The model under review builds one solid part; all positions refer to its coordinate system, in mm. Face numbers are marked on the shaded views. Round coordinates to 2 decimals unless told otherwise and drop trailing zeros. Order: outer loops, then holes, each group sorted by start corner. A loop starts at its lowest first (then second) coordinate and runs counter-clockwise, first axis right, second up. Notation, with made-up numbers: (37, 57.5) -> (51, 57.5) arc R12 cw to (51, 67.5) -> close; hole circle Ø6 at (63.5, 76). An arc over 180 degrees is marked (long way). Return JSON: item names as keys, results as strings. Group by question number.
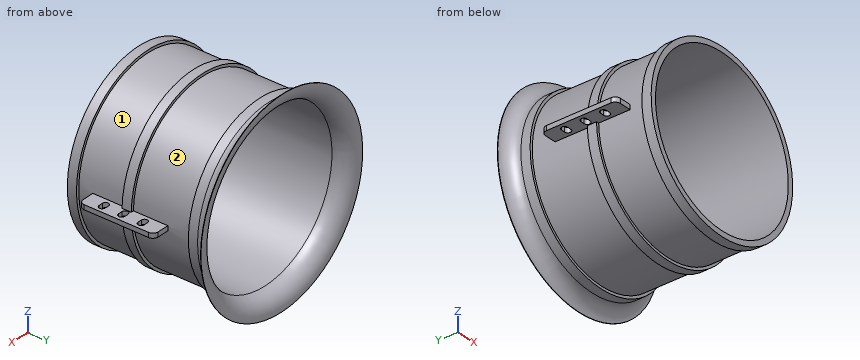
from build123d import *

# Parameters (mm, degrees)
BOSS_EXTRUDE1_DEPTH  = 1.325
FILLET1_R            = 3
FILLET1_OF_MIRROR1_R = 3


with BuildPart() as part:
    # Sketch2 → Revolve1 (revolve)
    with BuildSketch(Plane.XY, mode=Mode.PRIVATE) as revolve1_sk:
        with BuildLine():
            Line((46, 0), (46, 71.93668826))
            ThreePointArc((46, 71.93668826), (48.984023168, 78.718396784), (56, 81.1))
            Line((56, 81.1), (56, 80.9))
            ThreePointArc((56, 80.9), (51.02725979, 78.593132631), (49, 73.5))
            Line((49, 73.5), (49, 68.3))
            Line((49, 68.3), (47.5, 68.3))
            Line((47.5, 68.3), (47.5, 36.05))
            Line((47.5, 36.05), (49, 36.05))
            Line((49, 36.05), (49, 30.85))
            Line((49, 30.85), (47.5, 30.85))
            Line((47.5, 30.85), (47.5, 5.2))
            Line((47.5, 5.2), (49, 5.2))
            Line((49, 5.2), (49, 0))
            Line((49, 0), (46, 0))
        make_face()
    revolve(revolve1_sk.sketch.rotate(Axis((0, 0, 0), (0, 1, 0)), 90), axis=Axis((0, 0, 0), (0, 1, 0)))

    # Sketch3 → Boss-Extrude1 (add, symmetric)
    with BuildSketch(Plane.XY):
        Polygon((47.5, 55.45), (57.1, 55.45), (57.1, 13.15), (47.5, 13.15), (46, 13.15), (46, 55.45), align=None)
        with BuildLine():
            Line((51.15, 36.05), (53.45, 36.05))
            ThreePointArc((53.45, 36.05), (55.2, 34.3), (53.45, 32.55))
            Line((53.45, 32.55), (51.15, 32.55))
            ThreePointArc((51.15, 32.55), (49.4, 34.3), (51.15, 36.05))
        make_face(mode=Mode.SUBTRACT)
        with BuildLine():
            Line((51.15, 25.05), (53.45, 25.05))
            ThreePointArc((53.45, 25.05), (55.2, 23.3), (53.45, 21.55))
            Line((53.45, 21.55), (51.15, 21.55))
            ThreePointArc((51.15, 21.55), (49.4, 23.3), (51.15, 25.05))
        make_face(mode=Mode.SUBTRACT)
        with BuildLine():
            Line((51.15, 43.55), (53.45, 43.55))
            ThreePointArc((53.45, 43.55), (55.2, 45.3), (53.45, 47.05))
            Line((53.45, 47.05), (51.15, 47.05))
            ThreePointArc((51.15, 47.05), (49.4, 45.3), (51.15, 43.55))
        make_face(mode=Mode.SUBTRACT)
    boss_extrude1 = extrude(amount=BOSS_EXTRUDE1_DEPTH, both=True)

    # Fillet1
    fillet1_edges = [part.edges().sort_by_distance(p)[0] for p in [
        (57.1, 55.45, 0),
        (57.1, 13.15, 0),
    ]]
    fillet(fillet1_edges, radius=FILLET1_R)

    # Mirror1: Boss-Extrude1 across plane
    add(boss_extrude1.mirror(Plane(origin=(0, 0, 0), x_dir=(0, 0, 1), z_dir=(1, 0, 0))))

    # Fillet1 of Mirror1
    fillet1_of_mirror1_edges = [part.edges().sort_by_distance(p)[0] for p in [
        (-57.1, 55.45, 0),
        (-57.1, 13.15, 0),
    ]]
    fillet(fillet1_of_mirror1_edges, radius=FILLET1_OF_MIRROR1_R)


solid = part.part
Item 1: Wall thickness on line 1 along X through (y, z) = (35, 0); line 2 along X through (y, z) = (33, 0); line 3 along Z through (x, y) = (33.5, 34.5): over which ranges is each line inside the solid? List them lowest first.
Item 2: Insertion check: pin 1 Ø12 at (x, y) = (-34, 18.5) entering from -Z; pin 2 Ø2 at (x, z) = (-51, 0) entering from +Y; pin 3 Ø3 at (y, z) = (23.5, -7) entering from +X. Each pin has a flat end and moves straight along its axis. Give the tip position at first contact, or say it passes through.
Item 3: Consider section A-A on y = 34.3. State the section outline as (x, z) points (3 decimals), plus the area to 3 significant figures.
Item 4: The part is to be moulded in two halves that separate along Y. For the marked faces 1 and 2, say which applies: +Y half, -Y half, draft (parallel to the pull), parting line (faces both ways), or undercut.
Values:
{
 "1": {"line 1": "-57.1 to -55.05, -49.55 to -46, 46 to 49.55, 55.05 to 57.1", "line 2": "-57.1 to -54.62, -49.98 to -46, 46 to 49.98, 54.62 to 57.1", "line 3": "-35.76 to -31.52, 31.52 to 35.76"},
 "2": {"pin 1": "z = -38.37", "pin 2": "y = 80.56", "pin 3": "x = 47.18"},
 "3": {"outline": "(-57.1, -1.325) -> (-55.2, -1.325) -> (-55.2, 1.325) -> (-57.1, 1.325) -> close; (-49.4, -1.325) -> (-48.982, -1.325) arc R49 ccw to (48.982, -1.325) -> (49.4, -1.325) -> (49.4, 1.325) -> (48.982, 1.325) arc R49 ccw to (-48.982, 1.325) -> (-49.4, 1.325) -> close; (55.2, -1.325) -> (57.1, -1.325) -> (57.1, 1.325) -> (55.2, 1.325) -> close; hole circle Ø92 at (0, 0)", "area": "908 mm^2"},
 "4": {"face 1": "undercut", "face 2": "undercut"}
}
